from build123d import *

# Parameters (mm, degrees)
SKETCH3_R           = 1.7
BOSS_EXTRUDE2_DEPTH = 5
SKETCH8_R           = 1.7
BOSS_EXTRUDE4_DEPTH = 5
SKETCH10_R          = 2.75
CUT_EXTRUDE1_DEPTH  = 2.5


with BuildPart() as part:
    # Sketch3 → Boss-Extrude2 (new body)
    with BuildSketch(Plane(origin=(0, 0, 0), x_dir=(1, 0, 0), z_dir=(0, 1, 0))):
        with BuildLine():
            Line((-17.5, -12.5), (17.5, -12.5))
            ThreePointArc((17.5, -12.5), (21.035533906, -11.035533906), (22.5, -7.5))
            Line((22.5, -7.5), (22.5, 7.5))
            ThreePointArc((22.5, 7.5), (21.035533906, 11.035533906), (17.5, 12.5))
            Line((17.5, 12.5), (-17.5, 12.5))
            ThreePointArc((-17.5, 12.5), (-21.035533906, 11.035533906), (-22.5, 7.5))
            Line((-22.5, 7.5), (-22.5, -7.5))
            ThreePointArc((-22.5, -7.5), (-21.035533906, -11.035533906), (-17.5, -12.5))
        make_face()
        with Locations(Location((-15, 5, 0), (0, 0, 270))):
            Circle(SKETCH3_R, mode=Mode.SUBTRACT)
        with Locations(Location((15, 5, 0), (0, 0, 90))):
            Circle(SKETCH3_R, mode=Mode.SUBTRACT)
        with Locations(Location((15, -5, 0), (0, 0, 270))):
            Circle(SKETCH3_R, mode=Mode.SUBTRACT)
        with Locations(Location((-15, -5, 0), (0, 0, 90))):
            Circle(SKETCH3_R, mode=Mode.SUBTRACT)
    extrude(amount=BOSS_EXTRUDE2_DEPTH)

    # Sketch8 → Boss-Extrude4 (add, symmetric)
    with BuildSketch(Plane(origin=(0, 0, 0), x_dir=(0, 0, -1), z_dir=(1, 0, 0))):
        Polygon((-12.5, 5), (12.5, 5), (12.5, 40), (-24.442906699, 40), (-24.442906699, 16.942906699), align=None)
        with Locations((-16.758330249, 19.5)):
            Circle(SKETCH8_R, mode=Mode.SUBTRACT)
        with Locations((-12, 14.741669751)):
            Circle(SKETCH8_R, mode=Mode.SUBTRACT)
        with Locations((-5.5, 13)):
            Circle(SKETCH8_R, mode=Mode.SUBTRACT)
        with Locations((1, 14.741669751)):
            Circle(SKETCH8_R, mode=Mode.SUBTRACT)
        with Locations((5.758330249, 19.5)):
            Circle(SKETCH8_R, mode=Mode.SUBTRACT)
        with Locations((-18.5, 26)):
            Circle(SKETCH8_R, mode=Mode.SUBTRACT)
        with Locations((-16.758330249, 32.5)):
            Circle(SKETCH8_R, mode=Mode.SUBTRACT)
        with Locations((-5.5, 26)):
            Circle(SKETCH8_R, mode=Mode.SUBTRACT)
        with Locations((7.5, 26)):
            Circle(SKETCH8_R, mode=Mode.SUBTRACT)
        with Locations((5.758330249, 32.5)):
            Circle(SKETCH8_R, mode=Mode.SUBTRACT)
    extrude(amount=BOSS_EXTRUDE4_DEPTH, both=True)

    # Sketch10 → Cut-Extrude1 (cut)
    with BuildSketch(Plane(origin=(0, 5, 0), x_dir=(1, 0, 0), z_dir=(0, 1, 0))):
        with Locations(Location((15, -5, 0), (0, 0, 270))):
            Circle(SKETCH10_R)
        with Locations(Location((-15, -5, 0), (0, 0, 270))):
            Circle(SKETCH10_R)
        with Locations(Location((-15, 5, 0), (0, 0, 270))):
            Circle(SKETCH10_R)
        with Locations(Location((15, 5, 0), (0, 0, 270))):
            Circle(SKETCH10_R)
    extrude(amount=-CUT_EXTRUDE1_DEPTH, mode=Mode.SUBTRACT)


solid = part.part
Can you work these out from the model? Positions are in its coordinate system, mm. A direction names the side the tool comes from. Round coordinates to 2 decimals unless told otherwise and drop trailing zeros. Write each loop counter-clockwise with the first axis right and the second up, starting at its lowest first coordinate (ties: lowest second). Pieces come first, ordered by that corner, then holes. Notation, with made-up numbers: M 89,82.25 L 122,82.25 A17 cw 122,110.25 Z; hole C -5.5,11.25 d2. An arc over 180 degrees is marked long. Use a Markdown table: item, result.
Item 1: I want a section at C-C (x = -4). State how many separate pieces and enclosed holes the cut face has, and give its area (3 significant figures).
Found:
| item | result |
|---|---|
| separate pieces | 1 |
| enclosed holes | 10 |
| area | 1,260 mm2 |
Item 2: If I drill on line 1 along Y through (x, z) = (-1.25, 5.5); line 2 along Y through (x, z) = (-2.25, -1); line 3 along X through (y, z) = (20, 2.5), over which ranges is the centre line in solid material (lowest first)? Write a range as [from, to].
Found:
| item | result |
|---|---|
| line 1 | y = [0, 11.3], [14.7, 24.3], [27.7, 40] |
| line 2 | y = [0, 13.04], [16.44, 40] |
| line 3 | x = [-5, 5] |
Item 3: I want a section at A-A (z = -1). List the corners of the cut face in (x, y) for me, and give its area (3 significant figures).
Found:
| item | result |
|---|---|
| outline | M -22.5,0 L 22.5,0 L 22.5,5 L 5,5 L 5,13.04 L -5,13.04 L -5,5 L -22.5,5 Z; M -5,16.44 L 5,16.44 L 5,40 L -5,40 Z |
| area | 541 mm2 |
Item 4: We'd pull the mould along Z, two halves only. Please class faces 4 (the face through (0, 2, 12.5)), 5 (the face through (-0.07, 27.686, 5.721)), 6 (the face through (15, 2.5, -3)), 7 (the face through (-22.5, 2, 0)): released by +Z, released by -Z, zero draft, split by the parting line, or undercut.
Found:
| item | result |
|---|---|
| face 4 | released by +Z |
| face 5 | undercut |
| face 6 | undercut |
| face 7 | zero draft |
Item 5: For pin 1 Ø17.5 at (y, z) = (20, 6) entering from +X; pin 2 Ø1 at (x, z) = (-13.5, 13.5) entering from -Y; pin 3 Ø7 at (x, z) = (15, 5) entering from +Y; pin 4 Ø5.5 at (y, z) = (14.74, 12) entering from -X, each with a flat end and sliding along its axis, tell me the tip position at first contact or that it passes through.
Found:
| item | result |
|---|---|
| pin 1 | stops at x = 5 |
| pin 2 | passes through |
| pin 3 | stops at y = 5 |
| pin 4 | stops at x = -5 |
Item 6: I want a section at B-B (y = 32.5). List the corners of the cut face in (x, z) for me, and give its area (3 significant figures).
Found:
| item | result |
|---|---|
| outline | M -5,-12.5 L 5,-12.5 L 5,-7.46 L -5,-7.46 Z; M -5,-4.06 L 5,-4.06 L 5,15.06 L -5,15.06 Z; M -5,18.46 L 5,18.46 L 5,24.44 L -5,24.44 Z |
| area | 301 mm2 |
Item 7: Which directions (+Z, -Z, +X, -X, +Y, -Y) give clear straight access to the entire face, cutting with the end or side of a thin tool? Please do faces 1 (the face through (0.1, 11.1, 18.6)), 2 (the face through (-5, 23, 6)), 3 (the face through (17.727, 3.768, 4.642)).
Found:
| item | result |
|---|---|
| face 1 | +Z, +X, -X, -Y |
| face 2 | +Z, -Z, -X, +Y |
| face 3 | +Y |
